Part model, mm, in its own coordinate system. A direction names the side the tool comes from. Round coordinates to 2 decimals unless told otherwise and drop trailing zeros. Loops run counter-clockwise (first coordinate to the right, second up) from the corner with the lowest first, then second, coordinate; pieces in that order, holes last.
from build123d import *

# Parameters (mm, degrees)
SKETCH1_W           = 48.26
SKETCH1_H           = 25.5651
BOSS_EXTRUDE1_DEPTH = 17.78
SHELL1_T            = -2.54
SKETCH2_R           = 1.5875
BOSS_EXTRUDE2_DEPTH = 25.4
CUT_EXTRUDE1_DEPTH  = 12.7


with BuildPart() as part:
    # Sketch1 → Boss-Extrude1 (new, symmetric)
    with BuildSketch(Plane.XY):
        with Locations((24.13, -12.78255)):
            Rectangle(SKETCH1_W, SKETCH1_H)
    extrude(amount=BOSS_EXTRUDE1_DEPTH, both=True)

    # Shell1
    shell1_openings = [part.faces().sort_by_distance(p)[0] for p in [
        (24.13, -25.5651, 0),
    ]]
    offset(amount=SHELL1_T, openings=shell1_openings, kind=Kind.INTERSECTION)

    # Sketch2 → Boss-Extrude2 (add)
    with BuildSketch(Plane.XZ.offset(2.54)):
        with Locations(Location((10.16, 0, 0), (0, 0, 90))):
            Circle(SKETCH2_R)
    extrude(amount=BOSS_EXTRUDE2_DEPTH)

    # Sketch3 → Cut-Extrude1 (cut, symmetric)
    with BuildSketch(Plane.XY):
        Polygon((2.54, -25.5651), (2.54, -20.4851), (0, -20.4851), (0, -23.0251), (1.143, -23.0251), (0.508, -25.5651), align=None)
        Polygon((47.752, -25.5651), (47.117, -23.0251), (48.26, -23.0251), (48.26, -20.4851), (45.72, -20.4851), (45.72, -25.5651), align=None)
    extrude(amount=CUT_EXTRUDE1_DEPTH, both=True, mode=Mode.SUBTRACT)


solid = part.part
1) Slice it at C-C, the plane x = 13. Give the cut face in (y, z), then the cut area to 3 significant figures.
Values:
outline: (-25.57, -17.78) - (0, -17.78) - (0, 17.78) - (-25.57, 17.78) - (-25.57, 15.24) - (-2.54, 15.24) - (-2.54, -15.24) - (-25.57, -15.24) - close
area: 207 mm2
2) Tool access for faces 1 (the face through (48.26, -13, 0)), 2 (the face through (0.83, -24.28, -0.18)), 3 (the face through (46.7, -23, 12.7)): list every direction of +Z, -Z, +X, -X, +Y, -Y with a clear straight run to the whole face (end or side of a thin tool).
Values:
face 1: +Z, -Z, +X, +Y, -Y
face 2: -Y
face 3: none
3) Drop flat-ended pins along their axis: pin 1 Ø6 at (x, z) = (12, 8) entering from -Y; pin 2 Ø0.9 at (x, z) = (48, -2) entering from +Y. Give the stop position or say it passes through.
Values:
pin 1: stops at y = -2.54
pin 2: stops at y = 0
4) Wall check: line 1 along X through (y, z) = (-16.5, 0); line 2 along Z through (x, y) = (30.5, -13.75); line 3 along X through (y, z) = (-17.25, 14). Give the ranges that are in metal, low to high.
Values:
line 1: x = 0 to 2.54, 8.57 to 11.75, 45.72 to 48.26
line 2: z = -17.78 to -15.24, 15.24 to 17.78
line 3: x = 0 to 2.54, 45.72 to 48.26
5) Slice it at A-A, the plane z = 0. Give the cut face in (x, y), then the cut area to 3 significant figures.
Values:
outline: (0, -25.57) - (0.51, -25.57) - (1.14, -23.03) - (0, -23.03) - close; (0, -20.49) - (2.54, -20.49) - (2.54, -2.54) - (8.57, -2.54) - (8.57, -27.94) - (11.75, -27.94) - (11.75, -2.54) - (45.72, -2.54) - (45.72, -20.49) - (48.26, -20.49) - (48.26, 0) - (0, 0) - close; (47.12, -23.03) - (47.75, -25.57) - (48.26, -25.57) - (48.26, -23.03) - close
area: 299 mm2
6) Mould opens along Z. For faces 4 (the face through (2.54, -12, 0)), 5 (the face through (24, -25.565, 16)), 6 (the face through (24, -13, 17.78)) say: released by +Z, released by -Z, zero draft, split by the parting line, or undercut.
Values:
face 4: undercut
face 5: zero draft
face 6: released by +Z
7) Slice it at D-D, the plane z = 12. Give the cut face in (x, y).
Values:
outline: (0, -25.57) - (0.51, -25.57) - (1.14, -23.03) - (0, -23.03) - close; (0, -20.49) - (2.54, -20.49) - (2.54, -2.54) - (45.72, -2.54) - (45.72, -20.49) - (48.26, -20.49) - (48.26, 0) - (0, 0) - close; (47.12, -23.03) - (47.75, -25.57) - (48.26, -25.57) - (48.26, -23.03) - close
8) Slice it at B-B, the plane y = -4.25. Give the cut face in (x, z) (1 decimal), then the cut area to 3 significant figures.
Values:
outline: (0, -17.8) - (48.3, -17.8) - (48.3, 17.8) - (0, 17.8) - close; circle Ø3.2 at (10.2, 0); hole (2.5, -15.2) - (45.7, -15.2) - (45.7, 15.2) - (2.5, 15.2) - close
area: 408 mm2
